For this review, take the finished solid that the model builds, in its own axes (mm). A direction names the side the tool comes from. Round coordinates to 2 decimals unless told otherwise and drop trailing zeros. Order: outer loops, then holes, each group sorted by start corner. A loop starts at its lowest first (then second) coordinate and runs counter-clockwise, first axis right, second up. Notation, with made-up numbers: M 50.5,-4.5 L 95.5,-4.5 A30 cw 95.5,31.5 Z; hole C -23.5,55.5 d9. An arc over 180 degrees is marked long. Put each result on its own line as item: value.
from build123d import *

# Parameters (mm, degrees)
F0_W      = 100
F0_H      = 220
F1_DEPTH  = 40
F2_W      = 96
F2_H      = 216
F3_DEPTH  = 38
F5_R      = 2
F4_W      = 40
F4_H      = 30
F6_DEPTH  = 2
F8_W      = 5.3375530988
F8_H      = 25.0908638909
F9_DEPTH  = 10
F10_W     = 7.2876084596
F10_H     = 27.2723501176
F11_DEPTH = 10
F12_W     = 10
F12_H     = 7.1194600314
F13_DEPTH = 19.9
F14_W     = 9.5573319122
F14_H     = 8.1418789923
F15_DEPTH = 25
F16_W     = 5
F16_H     = 7.2876084596
F16_H_2   = 5.3375530988
F17_DEPTH = 15


with BuildPart() as f1:
    # F0 (on Top) → F1 (new body)
    with BuildSketch(Plane.XY):
        with Locations((-3.3097676933, 33.3972522417)):
            Rectangle(F0_W, F0_H)
    extrude(amount=F1_DEPTH)

    # F2 (on face) → F3 (cut)
    with BuildSketch(Plane.XY.offset(40)):
        with Locations((-3.3097676933, 33.3972522417)):
            Rectangle(F2_W, F2_H)
    extrude(amount=-F3_DEPTH, mode=Mode.SUBTRACT)

    # F5
    f5_edges = [f1.edges().sort_by_distance(p)[0] for p in [
        (-53.309768, -76.602748, 20),
        (46.690232, -76.602748, 20),
        (-53.309768, 143.397252, 20),
        (46.690232, 143.397252, 20),
    ]]
    fillet(f5_edges, radius=F5_R)

    # F4 (on face) → F6 (cut)
    with BuildSketch(Plane(origin=(-53.3097676933, 0, 0), x_dir=(0, -1, 0), z_dir=(-1, 0, 0))):
        with Locations((54.6027477583, 17)):
            Rectangle(F4_W, F4_H)
    extrude(amount=-F6_DEPTH, mode=Mode.SUBTRACT)

    # F8 (on face) → F9 (join)
    with BuildSketch(Plane.YZ.offset(46.6902323067)):
        with Locations((-6.6695250571, 27.4545680545)):
            Rectangle(F8_W, F8_H)
    extrude(amount=F9_DEPTH)

    # F10 (on face) → F11 (join)
    with BuildSketch(Plane.YZ.offset(46.6902323067)):
        with Locations((-29.5446543023, 26.3638249412)):
            Rectangle(F10_W, F10_H)
    extrude(amount=F11_DEPTH)

    # F12 (on face) → F13 (join)
    with BuildSketch(Plane(origin=(0, -25.9008500725, 0), x_dir=(-1, 0, 0), z_dir=(0, 1, 0))):
        with Locations((-51.6902323067, 16.2873798981)):
            Rectangle(F12_W, F12_H)
    extrude(amount=F13_DEPTH)

    # F14 (on face) → F15 (cut)
    with BuildSketch(Plane(origin=(44.6902323067, 0, 0), x_dir=(0, -1, 0), z_dir=(-1, 0, 0))):
        with Locations((17.3811190762, 31.3413348049)):
            Rectangle(F14_W, F14_H)
    extrude(amount=-F15_DEPTH, mode=Mode.SUBTRACT)

    # F16 (on face) → F17 (cut)
    with BuildSketch(Plane.XY.offset(40)):
        with Locations((49.1902323067, -29.5446543023)):
            Rectangle(F16_W, F16_H)
        with Locations((49.1902323067, -6.6695250571)):
            Rectangle(F16_W, F16_H_2)
    extrude(amount=-F17_DEPTH, mode=Mode.SUBTRACT)


solid = f1.part
(1) To check wall thickness, follow L1, parallel to X at y = 27, z = 17; L2, parallel to Y at x = -4.5, z = 36; L3, parallel to Z at x = -21, y = -29. State the ranges of each line that lie inside material, in increasing order.
A:
L1: x = -53.31 to -51.31, 44.69 to 46.69
L2: y = -76.6 to -74.6, 141.4 to 143.4
L3: z = 0 to 2
(2) Add section C-C on x = 21.5. Give the boundary of the cut face in (y, z), then the cut area to 3 significant figures.
A:
outline: M -76.6,0 L 143.4,0 L 143.4,40 L 141.4,40 L 141.4,2 L -74.6,2 L -74.6,40 L -76.6,40 Z
area: 592 mm2
(3) Insertion check: pin 1 Ø0.6 at (x, z) = (46, 29.5) entering from -Y; pin 2 Ø1.7 at (x, z) = (54, 14) entering from +Y; pin 3 Ø1 at (x, z) = (45.5, 31.5) entering from +Y. Each pin has a flat end and moves straight along its axis. Give the tip position at first contact, or say it passes through.
A:
pin 1: stops at y = -76.33
pin 2: stops at y = -6
pin 3: stops at y = 143.37
(4) Add section B-B on z = 8. Give the boundary of the cut face in (x, y).
A:
outline: M -53.31,-74.6 A2 ccw -51.31,-76.6 L 44.69,-76.6 A2 ccw 46.69,-74.6 L 46.69,141.4 A2 ccw 44.69,143.4 L -51.31,143.4 A2 ccw -53.31,141.4 L -53.31,-34.6 L -51.31,-34.6 L -51.31,141.4 L 44.69,141.4 L 44.69,-74.6 Z
(5) Draft analysis for pull direction X (two halves, no side actions). For faces 1 (the face through (54, -29, 40)), 2 (the face through (-4, 141.397, 21)), 3 (the face through (-53.31, 56, 20)), state which applies: released by +X, released by -X, zero draft, split by the parting line, or undercut.
A:
face 1: zero draft
face 2: undercut
face 3: released by -X
(6) For faces 4 (the face through (53, -4.001, 24)), 5 (the face through (53, -33.188, 23)), 6 (the face through (54, -25.901, 28)), 7 (the face through (51.69, -7, 33)), list the 3-axis set-ups (+Z, -Z, +X, -X, +Y, -Y) from which the entire face can be reached by the end or side of a thin tool; tool diameter is ignored.
A:
face 4: +Z, -Z, +X, +Y
face 5: +Z, -Z, +X, -Y
face 6: +Z, +X
face 7: +Z, +Y, -Y
(7) Add section A-A on y = -48. Give the boundary of the cut face in (x, z), then the cut area to 3 significant figures.
A:
outline: M -53.31,0 L 46.69,0 L 46.69,40 L 44.69,40 L 44.69,2 L -53.31,2 Z; M -53.31,32 L -51.31,32 L -51.31,40 L -53.31,40 Z
area: 292 mm2
(8) Add section D-D on y = 99. Give the boundary of the cut face in (x, z), then the cut area to 3 significant figures.
A:
outline: M -53.31,0 L 46.69,0 L 46.69,40 L 44.69,40 L 44.69,2 L -51.31,2 L -51.31,40 L -53.31,40 Z
area: 352 mm2
